Geometry check sheet. Reference: drawing and pictorial views, mm from the part's lowest x, y, z. A direction names the side the tool comes from. Round coordinates to 2 decimals unless told otherwise and drop trailing zeros. Write each loop counter-clockwise with the first axis right and the second up, starting at its lowest first coordinate (ties: lowest second). Pieces come first, ordered by that corner, then holes.
Item 1: Depth check by flat-ended pin: pin 1 (2 mm diameter, centred on x = 27, y = 30.5, fed in from -Z); pin 2 (8 mm diameter, centred on y = 17.5, z = 8.5, fed in from +X); pin 3 (3 mm diameter, centred on x = 8, z = 22.5, fed in from +Y) (3 decimals). Enter the tip coordinate at first touch or a pass-through.
Item 2: Section check B-B, the plane x = 12. Record the cut outline in (y, z) (1 decimal).
Item 3: Section check A-A, the plane y = 9.5. Record the cut outline in (x, z) (1 decimal), plus the area to 3 significant figures.
Item 4: Section check D-D, the plane z = 23. Record the cut outline in (x, y) (1 decimal).
Item 5: Material ranges on line 1 along Z through (x, y) = (22.5, 14) (1 decimal); line 2 along Y through (x, z) = (22, 18.5) (1 decimal), recorded low to high.
Item 6: Set-up check for the marked faces 1 and 2: record each of +Z, -Z, +X, -X, +Y, -Y from which the full face is reachable in a straight line by a thin tool's end or side.
Item 7: Release check for a two-part mould opening along Z. For the marked faces 3, 4 and 5 record: pulls with the +Z half, pulls with the -Z half, needs draft (parallel to the pull), parting line crosses it, or undercut.
Item 8: Section check C-C, the plane y = 28. Record the cut outline in (x, z) (1 decimal), plus the area to 3 significant figures.
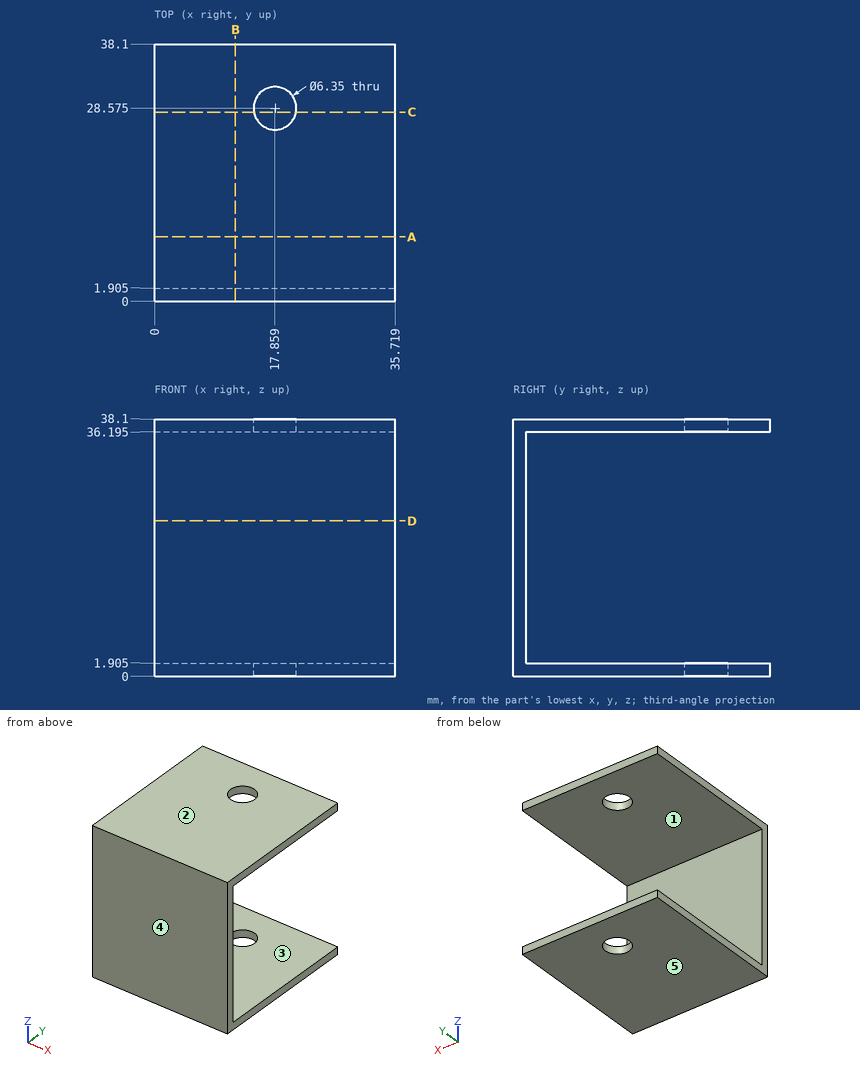
Values found:
1. pin 1: stops at z = 0
1. pin 2: passes through
1. pin 3: stops at y = 1.905
2. outline: (0, 0) - (38.1, 0) - (38.1, 1.9) - (1.9, 1.9) - (1.9, 36.2) - (38.1, 36.2) - (38.1, 38.1) - (0, 38.1) - close
3. outline: (0, 0) - (35.7, 0) - (35.7, 1.9) - (0, 1.9) - close; (0, 36.2) - (35.7, 36.2) - (35.7, 38.1) - (0, 38.1) - close
3. area: 136 mm2
4. outline: (0, 0) - (35.7, 0) - (35.7, 1.9) - (0, 1.9) - close
5. line 1: z = 0 to 1.9, 36.2 to 38.1
5. line 2: y = 0 to 1.9
6. face 1: +X, -X, +Y
6. face 2: +Z, +X, -X, +Y, -Y
7. face 3: undercut
7. face 4: needs draft
7. face 5: pulls with the -Z half
8. outline: (0, 0) - (14.7, 0) - (14.7, 1.9) - (0, 1.9) - close; (0, 36.2) - (14.7, 36.2) - (14.7, 38.1) - (0, 38.1) - close; (21, 0) - (35.7, 0) - (35.7, 1.9) - (21, 1.9) - close; (21, 36.2) - (35.7, 36.2) - (35.7, 38.1) - (21, 38.1) - close
8. area: 112 mm2
